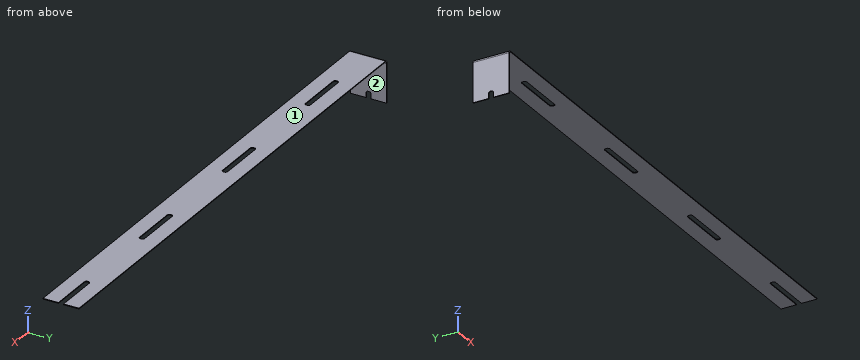
```python
from build123d import *

# Parameters (mm, degrees)
F0_W     = 4
F0_H     = 3
F1_DEPTH = 0.15
F2_DEPTH = 1.9
F3_W     = 0.15
F3_H     = 7
F4_DEPTH = 8
F6_DEPTH = 25
F7_R     = 0.5


with BuildPart() as f1:
    # F0 (on Top) → F1 (new body)
    with BuildSketch(Plane.XY):
        with BuildLine():
            Line((0, 3.5), (0, -3.5))
            Line((0, -3.5), (13.775, -3.5))
            Line((13.775, -3.5), (13.775, -0.5))
            Line((13.775, -0.5), (9.175, -0.5))
            ThreePointArc((9.175, -0.5), (8.8921572875, -0.3828427125), (8.775, -0.1))
            Line((8.775, -0.1), (8.775, 0.1))
            ThreePointArc((8.775, 0.1), (8.8921572875, 0.3828427125), (9.175, 0.5))
            Line((9.175, 0.5), (13.775, 0.5))
            Line((13.775, 0.5), (13.775, 3.5))
            Line((13.775, 3.5), (0, 3.5))
        make_face()
        with BuildLine():
            Line((13.775, -0.5), (13.775, -3.5))
            Line((13.775, -3.5), (27.55, -3.5))
            Line((27.55, -3.5), (41.325, -3.5))
            Line((41.325, -3.5), (41.325, -0.5))
            Line((41.325, -0.5), (36.725, -0.5))
            ThreePointArc((36.725, -0.5), (36.4421572875, -0.3828427125), (36.325, -0.1))
            Line((36.325, -0.1), (36.325, 0.1))
            ThreePointArc((36.325, 0.1), (36.4421572875, 0.3828427125), (36.725, 0.5))
            Line((36.725, 0.5), (41.325, 0.5))
            Line((41.325, 0.5), (41.325, 3.5))
            Line((41.325, 3.5), (27.55, 3.5))
            Line((27.55, 3.5), (13.775, 3.5))
            Line((13.775, 3.5), (13.775, 0.5))
            Line((13.775, 0.5), (18.375, 0.5))
            ThreePointArc((18.375, 0.5), (18.6578427125, 0.3828427125), (18.775, 0.1))
            Line((18.775, 0.1), (18.775, -0.1))
            ThreePointArc((18.775, -0.1), (18.6578427125, -0.3828427125), (18.375, -0.5))
            Line((18.375, -0.5), (13.775, -0.5))
        make_face()
        with BuildLine():
            Line((41.325, -0.5), (41.325, -3.5))
            Line((41.325, -3.5), (55.1, -3.5))
            Line((55.1, -3.5), (68.875, -3.5))
            Line((68.875, -3.5), (68.875, -0.5))
            Line((68.875, -0.5), (64.275, -0.5))
            ThreePointArc((64.275, -0.5), (63.9921572875, -0.3828427125), (63.875, -0.1))
            Line((63.875, -0.1), (63.875, 0.1))
            ThreePointArc((63.875, 0.1), (63.9921572875, 0.3828427125), (64.275, 0.5))
            Line((64.275, 0.5), (68.875, 0.5))
            Line((68.875, 0.5), (68.875, 3.5))
            Line((68.875, 3.5), (55.1, 3.5))
            Line((55.1, 3.5), (41.325, 3.5))
            Line((41.325, 3.5), (41.325, 0.5))
            Line((41.325, 0.5), (45.925, 0.5))
            ThreePointArc((45.925, 0.5), (46.2078427125, 0.3828427125), (46.325, 0.1))
            Line((46.325, 0.1), (46.325, -0.1))
            ThreePointArc((46.325, -0.1), (46.2078427125, -0.3828427125), (45.925, -0.5))
            Line((45.925, -0.5), (41.325, -0.5))
        make_face()
        with BuildLine():
            Line((68.875, -0.5), (68.875, -3.5))
            Line((68.875, -3.5), (82.65, -3.5))
            Line((82.65, -3.5), (96.425, -3.5))
            Line((96.425, -3.5), (96.425, -0.5))
            Line((96.425, -0.5), (91.825, -0.5))
            ThreePointArc((91.825, -0.5), (91.5421572875, -0.3828427125), (91.425, -0.1))
            Line((91.425, -0.1), (91.425, 0.1))
            ThreePointArc((91.425, 0.1), (91.5421572875, 0.3828427125), (91.825, 0.5))
            Line((91.825, 0.5), (96.425, 0.5))
            Line((96.425, 0.5), (96.425, 3.5))
            Line((96.425, 3.5), (82.65, 3.5))
            Line((82.65, 3.5), (68.875, 3.5))
            Line((68.875, 3.5), (68.875, 0.5))
            Line((68.875, 0.5), (73.475, 0.5))
            ThreePointArc((73.475, 0.5), (73.7578427125, 0.3828427125), (73.875, 0.1))
            Line((73.875, 0.1), (73.875, -0.1))
            ThreePointArc((73.875, -0.1), (73.7578427125, -0.3828427125), (73.475, -0.5))
            Line((73.475, -0.5), (68.875, -0.5))
        make_face()
        with Locations((98.425, -2)):
            Rectangle(F0_W, F0_H)
        with Locations((98.425, 2)):
            Rectangle(F0_W, F0_H)
    extrude(amount=F1_DEPTH)

    # F2 (add): a face of the model
    f2_faces = [f1.faces().sort_by_distance(p)[0] for p in [
        (0, 0, 0.075),
    ]]
    extrude(f2_faces, amount=F2_DEPTH)

    # F3 (on face) → F4 (join)
    with BuildSketch(Plane(origin=(0, 0, 0), x_dir=(1, 0, 0), z_dir=(0, 0, -1))):
        with Locations((-1.825, 0)):
            Rectangle(F3_W, F3_H)
    extrude(amount=F4_DEPTH)

    # F5 (on face) → F6 (cut)
    with BuildSketch(Plane(origin=(-1.9, 0, 0), x_dir=(0, -1, 0), z_dir=(-1, 0, 0))):
        with BuildLine():
            ThreePointArc((0.5, -7.1), (0.3828427125, -6.8171572875), (0.1, -6.7))
            Line((0.1, -6.7), (-0.1, -6.7))
            ThreePointArc((-0.1, -6.7), (-0.3828427125, -6.8171572875), (-0.5, -7.1))
            Line((-0.5, -7.1), (-0.5, -8))
            Line((-0.5, -8), (0.5, -8))
            Line((0.5, -8), (0.5, -7.1))
        make_face()
    extrude(amount=-F6_DEPTH, mode=Mode.SUBTRACT)

    # F7
    f7_edges = [f1.edges().sort_by_distance(p)[0] for p in [
        (-1.9, 0, 0.15),
        (-1.75, 0, 0),
    ]]
    fillet(f7_edges, radius=F7_R)


solid = f1.part
```
Could you check a few things on this model? Use its own coordinates, in mm. Face numbers are marked on the shaded views. A direction names the side the tool comes from. Coordinates: 2 decimals unless noted, no trailing zeros. Write each loop counter-clockwise with the first axis right and the second up, starting at its lowest first coordinate (ties: lowest second). Pieces come first, ordered by that corner, then holes. Notation, with made-up numbers: (3.5, -26.75) -> (52.5, -26.75) arc R19 ccw to (52.5, -19.75) -> close; hole circle Ø5 at (35, 2). An arc over 180 degrees is marked (long way). Write item = value, one per line. Start each with the question number.
(1) I want a section at D-D (z = -4.5). Please give me the cut outline in (x, y), plus the area to 3 significant figures.
(2) I want a section at B-B (y = -1.75). Please give me the cut outline in (x, z) (3 decimals), plus the area to 3 significant figures.
(3) I want a section at A-A (x = 66). Please give me the cut outline in (y, z).
(4) Which directions (+Z, -Z, +X, -X, +Y, -Y) give clear straight access to the entire face, cutting with the end or side of a thin tool? Please do the marked faces 1 and 2.
(5) Will this pin go through, and if not, where does the flat tip stop? pin 1 (3.5 mm diameter, centred on y = 0.5, z = -4, fed in from +X).
(6) I need wall thicknesses on line 1 (Z direction, x = 62, y = 0.75); line 2 (X direction, y = 0.25, z = -0.25). Which ranges of each line are inside material? Lowest first, please. Write a range as [from, to].
(7) I want a section at C-C (x = 49). Please give me the cut outline in (y, z).
Result set:
q1.outline = (-1.9, -3.5) -> (-1.75, -3.5) -> (-1.75, 3.5) -> (-1.9, 3.5) -> close
q1.area = 1.05 mm2
q2.outline = (-1.9, -8) -> (-1.75, -8) -> (-1.75, -0.5) arc R0.5 cw to (-1.25, 0) -> (100.425, 0) -> (100.425, 0.15) -> (-1.4, 0.15) arc R0.5 ccw to (-1.9, -0.35) -> close
q2.area = 16.5 mm2
q3.outline = (-3.5, 0) -> (-0.5, 0) -> (-0.5, 0.15) -> (-3.5, 0.15) -> close; (0.5, 0) -> (3.5, 0) -> (3.5, 0.15) -> (0.5, 0.15) -> close
q4.face_1 = +Z, +X, -X, +Y, -Y
q4.face_2 = -Z, +X, +Y, -Y
q5.pin_1 = -1.75
q6.line_1 = [0, 0.15]
q6.line_2 = [-1.89, -1.68]
q7.outline = (-3.5, 0) -> (3.5, 0) -> (3.5, 0.15) -> (-3.5, 0.15) -> close
